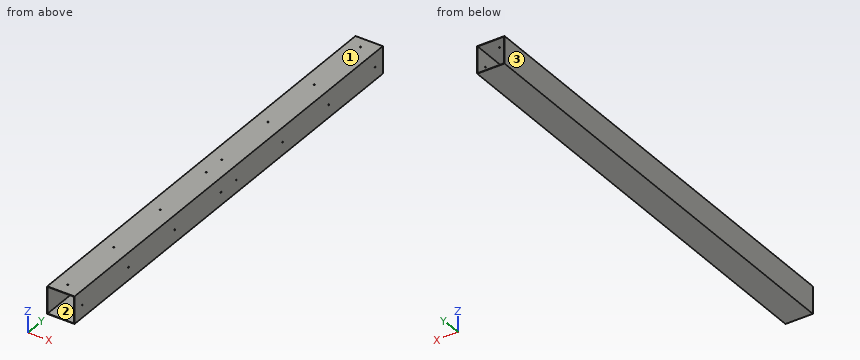
```python
from build123d import *

# Parameters (mm, degrees)
SKETCH_1_W          = 120
SKETCH_1_H          = 120
SKETCH_1_W_2        = 116
SKETCH_1_H_2        = 116
EXTRUDE_1_DEPTH     = 2000
SKETCH_2_R          = 2.5
CUT_EXTRUDE_1_DEPTH = 2002.799190728
SKETCH_3_R          = 2.5
CUT_EXTRUDE_2_DEPTH = 2002.799190728


with BuildPart() as part:
    # 草图1 → 拉伸-薄壁1 (new body)
    with BuildSketch(Plane(origin=(0, 0, 0), x_dir=(1, 0, 0), z_dir=(0, 1, 0))):
        Rectangle(SKETCH_1_W, SKETCH_1_H)
        Rectangle(SKETCH_1_W_2, SKETCH_1_H_2, mode=Mode.SUBTRACT)
    extrude(amount=EXTRUDE_1_DEPTH)

    # 草图2 → 切除-拉伸1 (cut, through all)
    with BuildSketch(Plane(origin=(0, 0, 0), x_dir=(0, 0, -1), z_dir=(1, 0, 0))):
        with Locations(Location((4, 50, 0), (0, 0, 180))):
            Circle(SKETCH_2_R)
        with Locations(Location((4, 350, 0), (0, 0, 180))):
            Circle(SKETCH_2_R)
        with Locations(Location((4, 650, 0), (0, 0, 180))):
            Circle(SKETCH_2_R)
        with Locations(Location((4, 950, 0), (0, 0, 180))):
            Circle(SKETCH_2_R)
        with Locations(Location((4, 1950, 0), (0, 0, 180))):
            Circle(SKETCH_2_R)
        with Locations(Location((4, 1650, 0), (0, 0, 180))):
            Circle(SKETCH_2_R)
        with Locations(Location((4, 1350, 0), (0, 0, 180))):
            Circle(SKETCH_2_R)
        with Locations(Location((4, 1050, 0), (0, 0, 180))):
            Circle(SKETCH_2_R)
    extrude(amount=CUT_EXTRUDE_1_DEPTH, mode=Mode.SUBTRACT)

    # 草图3 → 切除-拉伸2 (cut, through all)
    with BuildSketch(Plane.XY):
        with Locations(Location((-4, 50, 0), (0, 0, 180))):
            Circle(SKETCH_3_R)
        with Locations(Location((-4, 350, 0), (0, 0, 180))):
            Circle(SKETCH_3_R)
        with Locations(Location((-4, 650, 0), (0, 0, 180))):
            Circle(SKETCH_3_R)
        with Locations(Location((-4, 950, 0), (0, 0, 180))):
            Circle(SKETCH_3_R)
        with Locations(Location((-4, 1950, 0), (0, 0, 180))):
            Circle(SKETCH_3_R)
        with Locations(Location((-4, 1650, 0), (0, 0, 180))):
            Circle(SKETCH_3_R)
        with Locations(Location((-4, 1350, 0), (0, 0, 180))):
            Circle(SKETCH_3_R)
        with Locations(Location((-4, 1050, 0), (0, 0, 180))):
            Circle(SKETCH_3_R)
    extrude(amount=CUT_EXTRUDE_2_DEPTH, mode=Mode.SUBTRACT)


solid = part.part
```
Can you work these out from the model? Positions are in its coordinate system, mm. Face numbers are marked on the shaded views. Coordinates: 2 decimals unless noted, no trailing zeros. Order: outer loops, then holes, each group sorted by start corner. A loop starts at its lowest first (then second) coordinate and runs counter-clockwise, first axis right, second up. Notation, with made-up numbers: (3.5, 18.5) - (44.5, 18.5) arc R20 ccw to (44.5, 57.5) - close; hole circle Ø11 at (20.5, 14.5). An arc over 180 degrees is marked (long way). Answer in a Markdown table with one row per item.
1. Suppose I cut it at B-B (y = 307). Please give me the cut outline in (x, z), and give its area (3 significant figures).
Reply:
| item | result |
|---|---|
| outline | (-60, -60) - (60, -60) - (60, 60) - (-60, 60) - close; hole (-58, -58) - (58, -58) - (58, 58) - (-58, 58) - close |
| area | 944 mm^2 |
2. If we mould it in two halves opening along X, with no side actions, what happens to the marked faces 1, 2 and 3? For each: pulls with the +X half, pulls with the -X half, needs draft (parallel to the pull), parting line crosses it, or undercut.
Reply:
| item | result |
|---|---|
| face 1 | needs draft |
| face 2 | undercut |
| face 3 | pulls with the -X half |
3. Suppose I cut it at C-C (z = 20). Please give me the cut outline in (x, y), and give its area (3 significant figures).
Reply:
| item | result |
|---|---|
| outline | (-60, 0) - (-58, 0) - (-58, 2000) - (-60, 2000) - close; (58, 0) - (60, 0) - (60, 2000) - (58, 2000) - close |
| area | 8,000 mm^2 |
4. If I drill on line 1 along X through (y, z) = (318, -50); line 2 along Z through (x, y) = (59.1, 1650), over which ranges is the centre line in solid material (lowest first)?
Reply:
| item | result |
|---|---|
| line 1 | x = -60 to -58, 58 to 60 |
| line 2 | z = -60 to -6.5, -1.5 to 60 |
5. For pin 1 (4 mm diameter, centred on y = 50, z = -4, fed in from +X); pin 2 (3 mm diameter, centred on x = -4, y = 50, fed in from +Z), each with a flat end and sliding along its axis, tell me the tip position at first contact or that it passes through.
Reply:
| item | result |
|---|---|
| pin 1 | stops at x = -58 |
| pin 2 | stops at z = -58 |
6. Suppose I cut it at A-A (x = 41.5). Please give me the cut outline in (y, z).
Reply:
| item | result |
|---|---|
| outline | (0, -60) - (2000, -60) - (2000, -58) - (0, -58) - close; (0, 58) - (2000, 58) - (2000, 60) - (0, 60) - close |
